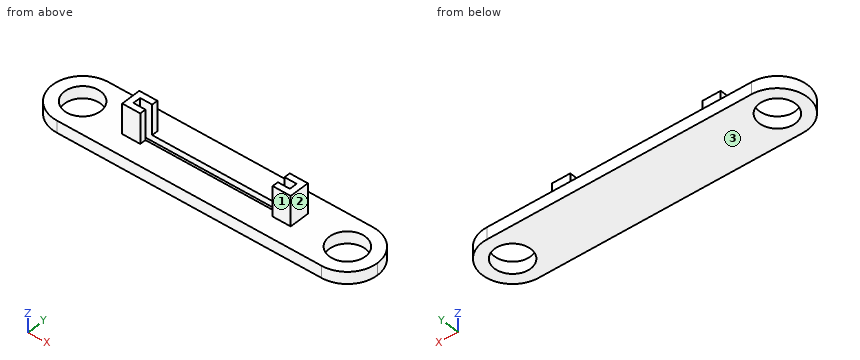
```python
from build123d import *

# Parameters (mm, degrees)
F0_R     = 3
F1_DEPTH = 2
F3_DEPTH = 5
F2_W     = 11
F2_H     = 0.65
F2_W_2   = 2
F4_DEPTH = 1


with BuildPart() as f1:
    # F0 (on Top) → F1 (new body)
    with BuildSketch(Plane.XY):
        with BuildLine():
            ThreePointArc((31.2996847679, -5), (26.2996847679, 0), (31.2996847679, 5))
            Line((31.2996847679, 5), (-12.7003152321, 5))
            ThreePointArc((-12.7003152321, 5), (-9.1647813261, 3.5355339059), (-7.7003152321, 0))
            ThreePointArc((-7.7003152321, 0), (-9.1647813261, -3.5355339059), (-12.7003152321, -5))
            Line((-12.7003152321, -5), (31.2996847679, -5))
        make_face()
        with BuildLine():
            ThreePointArc((-7.7003152321, 0), (-9.1647813261, 3.5355339059), (-12.7003152321, 5))
            ThreePointArc((-12.7003152321, 5), (-17.7003152321, 0), (-12.7003152321, -5))
            ThreePointArc((-12.7003152321, -5), (-9.1647813261, -3.5355339059), (-7.7003152321, 0))
        make_face()
        with Locations((-12.7003152321, 0)):
            Circle(F0_R, mode=Mode.SUBTRACT)
        with BuildLine():
            ThreePointArc((31.2996847679, -5), (34.8352186739, -3.5355339059), (36.2996847679, 0))
            ThreePointArc((36.2996847679, 0), (34.8352186739, 3.5355339059), (31.2996847679, 5))
            ThreePointArc((31.2996847679, 5), (26.2996847679, 0), (31.2996847679, -5))
        make_face()
        with Locations((31.2996847679, 0)):
            Circle(F0_R, mode=Mode.SUBTRACT)
    extrude(amount=F1_DEPTH)

    # F2 (on face) → F3 (join)
    with BuildSketch(Plane.XY.offset(2)):
        Polygon((-3.7003152321, 0), (-4.7003152321, 0), (-4.7003152321, -1.65), (-1.7003152321, -1.65), (-1.7003152321, -0.65), (-3.7003152321, -0.65), align=None)
        Polygon((-1.7003152321, 0.65), (-1.7003152321, 1.65), (-4.7003152321, 1.65), (-4.7003152321, 0), (-3.7003152321, 0), (-3.7003152321, 0.65), align=None)
        Polygon((23.2996847679, 1.65), (20.2996847679, 1.65), (20.2996847679, 0.65), (22.2996847679, 0.65), (22.2996847679, 0), (23.2996847679, 0), align=None)
        Polygon((23.2996847679, -1.65), (23.2996847679, 0), (22.2996847679, 0), (22.2996847679, -0.65), (20.2996847679, -0.65), (20.2996847679, -1.65), align=None)
    extrude(amount=F3_DEPTH)

    # F2 (on face) → F4 (cut)
    with BuildSketch(Plane.XY.offset(2)):
        with Locations((3.7996847679, -0.325)):
            Rectangle(F2_W, F2_H)
        with Locations((3.7996847679, 0.325)):
            Rectangle(F2_W, F2_H)
        with Locations((-2.7003152321, -0.325)):
            Rectangle(F2_W_2, F2_H)
        with Locations((-2.7003152321, 0.325)):
            Rectangle(F2_W_2, F2_H)
        with Locations((14.7996847679, -0.325)):
            Rectangle(F2_W, F2_H)
        with Locations((14.7996847679, 0.325)):
            Rectangle(F2_W, F2_H)
        with Locations((21.2996847679, -0.325)):
            Rectangle(F2_W_2, F2_H)
        with Locations((21.2996847679, 0.325)):
            Rectangle(F2_W_2, F2_H)
    extrude(amount=-F4_DEPTH, mode=Mode.SUBTRACT)


solid = f1.part
```
The listing builds one solid part. Answer for the finished solid, in the listing's coordinates (mm). Face numbers are marked on the shaded views. A direction names the side the tool comes from. Give positions to 0.01 mm unless a question says otherwise; leave off trailing zeros. Order: outer loops, then holes, each group sorted by start corner. A loop starts at its lowest first (then second) coordinate and runs counter-clockwise, first axis right, second up. Notation, with made-up numbers: (-29, 18) -> (13, 18) arc R25 ccw to (13, 39) -> close; hole circle Ø9 at (9.25, 74.5). An arc over 180 degrees is marked (long way). Answer as a JSON object with one key per item and string values. Group by question number.
Item 1: Flat-ended cylindrical pins translate along their axes: pin 1 (0.8 mm diameter, centred on y = -1, z = 5, fed in from -X); pin 2 (2.5 mm diameter, centred on x = 22, z = 4.5, fed in from -Y); pin 3 (2.5 mm diameter, centred on y = -0.5, z = 5.5, fed in from +X). Find the tip coordinate at first contact, or state that the pin passes through.
Item 2: The part is cut by section B-B on y = 2.25. Write down the section's boundary in (x, z).
Item 3: The part is cut by section D-D on x = 0.5. Write down the section's boundary in (y, z).
Item 4: Consider L1, parallel to Y at x = 10, z = 1.25; L2, parallel to X at y = -1.5, z = 5.25; L3, parallel to X at y = -1, z = 1.25. Determine where each line is inside the solid, lowest interval first. Write a range as from..to.
Item 5: The part is cut by section C-C on x = -10.5. Write down the section's boundary in (y, z), and give its area (3 significant figures).
Item 6: The part is cut by section A-A on z = 5.5. Write down the section's boundary in (x, y), and give its area (3 significant figures).
Item 7: A tool of negligible diameter and unlimited length cuts with its end or side. For the marked faces 1, 2 and 3, from which of +Z, -Z, +X, -X, +Y, -Y can it reach the whole face along a straight path? Write none if from no direction.
Result set:
{
 "1": {"pin 1": "x = -4.7", "pin 2": "y = -1.65", "pin 3": "x = 23.3"},
 "2": {"outline": "(-17.17, 0) -> (-14.68, 0) -> (-14.68, 2) -> (-17.17, 2) -> close; (-10.72, 0) -> (29.32, 0) -> (29.32, 2) -> (-10.72, 2) -> close; (33.28, 0) -> (35.76, 0) -> (35.76, 2) -> (33.28, 2) -> close"},
 "3": {"outline": "(-5, 0) -> (5, 0) -> (5, 2) -> (0.65, 2) -> (0.65, 1) -> (-0.65, 1) -> (-0.65, 2) -> (-5, 2) -> close"},
 "4": {"L1": "-5..-0.65, 0.65..5", "L2": "-4.7..-1.7, 20.3..23.3", "L3": "-17.6..-15.53, -9.87..28.47, 34.13..36.2"},
 "5": {"outline": "(-5, 0) -> (-2.04, 0) -> (-2.04, 2) -> (-5, 2) -> close; (2.04, 0) -> (5, 0) -> (5, 2) -> (2.04, 2) -> close", "area": "11.8 mm²"},
 "6": {"outline": "(-4.7, -1.65) -> (-1.7, -1.65) -> (-1.7, -0.65) -> (-3.7, -0.65) -> (-3.7, 0.65) -> (-1.7, 0.65) -> (-1.7, 1.65) -> (-4.7, 1.65) -> close; (20.3, -1.65) -> (23.3, -1.65) -> (23.3, 1.65) -> (20.3, 1.65) -> (20.3, 0.65) -> (22.3, 0.65) -> (22.3, -0.65) -> (20.3, -0.65) -> close", "area": "14.6 mm²"},
 "7": {"face 1": "+Z, +X, -X, -Y", "face 2": "+Z, +X, +Y, -Y", "face 3": "-Z, +X, -X, +Y, -Y"}
}
